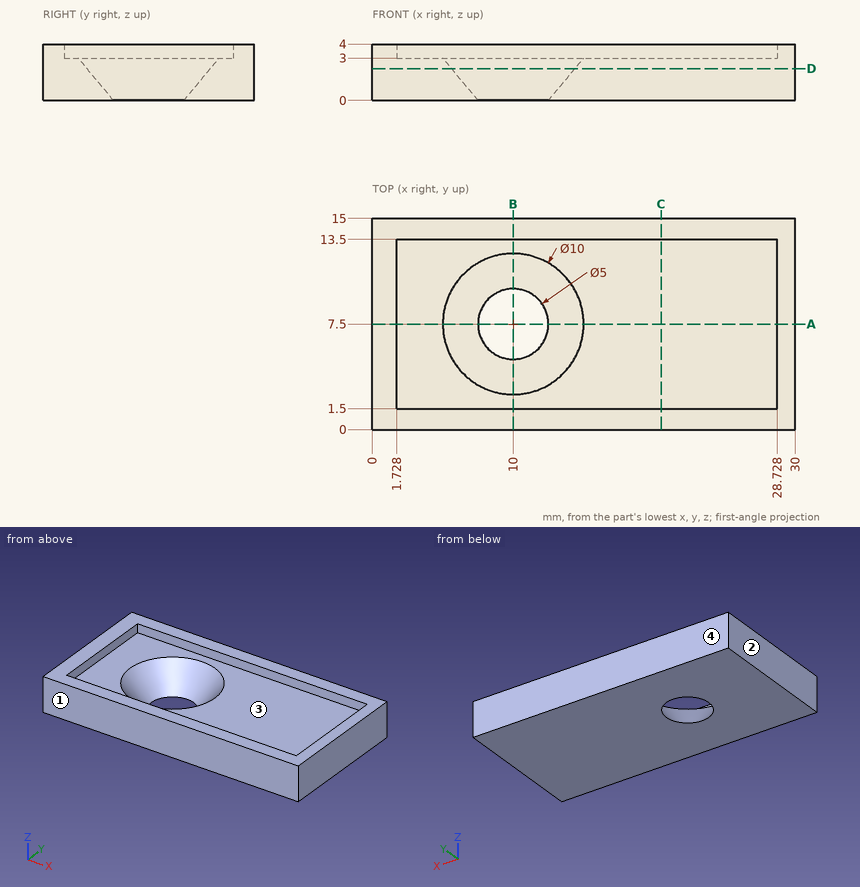
Geometry: see drawing. Coordinates: mm, zero at the bounding-box minimum. Give positions to 0.01 mm unless a question says otherwise; leave off trailing zeros. Order: outer loops, then holes, each group sorted by start corner. A loop starts at its lowest first (then second) coordinate and runs counter-clockwise, first axis right, second up. Notation, with made-up numbers: (77.5, -17) - (112.5, -17) arc R17 ccw to (112.5, 12) - close; hole circle Ø2 at (-22, 54.5). An arc over 180 degrees is marked (long way). Use CSV: the item, a comma, the result in double quotes.
1. Mould query, pull axis Y, two halves, no side actions, for the marked faces 1, 2, 3 and 4. Classes: +Y half, -Y half, draft (parallel to the pull), parting line (faces both ways), or undercut.
Answers below:
face 1,"-Y half"
face 2,"draft"
face 3,"undercut"
face 4,"+Y half"
2. Material intervals for line 1 along Y through (x, z) = (3.75, 3.4); line 2 along X through (y, z) = (9.5, 3.45); line 3 along Z through (x, y) = (27.25, 6.5), sorted ascending. Write a range as from..to.
Answers below:
line 1,"0..1.5, 13.5..15"
line 2,"0..1.73, 28.73..30"
line 3,"0..3"
3. Section query B-B (x = 10). Output: boundary loops of the cut face in (y, z), plus the area to 3 significant figures.
Answers below:
outline,"(0, 0) - (5, 0) - (2.5, 3) - (1.5, 3) - (1.5, 4) - (0, 4) - close; (10, 0) - (15, 0) - (15, 4) - (13.5, 4) - (13.5, 3) - (12.5, 3) - close"
area,"25.5 mm2"
4. Section query A-A (y = 7.5). Output: boundary loops of the cut face in (x, z).
Answers below:
outline,"(0, 0) - (7.5, 0) - (5, 3) - (1.73, 3) - (1.73, 4) - (0, 4) - close; (12.5, 0) - (30, 0) - (30, 4) - (28.73, 4) - (28.73, 3) - (15, 3) - close"
5. Section query C-C (x = 20.5). Output: boundary loops of the cut face in (y, z).
Answers below:
outline,"(0, 0) - (15, 0) - (15, 4) - (13.5, 4) - (13.5, 3) - (1.5, 3) - (1.5, 4) - (0, 4) - close"
6. Section query D-D (z = 2.25). Output: boundary loops of the cut face in (x, y) (3 decimals), plus the area to 3 significant figures.
Answers below:
outline,"(0, 0) - (30, 0) - (30, 15) - (0, 15) - close; hole circle Ø8.75 at (10, 7.5)"
area,"390 mm2"
7. Contact query for a flat-ended pin moving along its axis: pin 1 (3 mm diameter, centred on x = 16, y = 11, fed in from +Z). Output: stop coordinate, or through.
Answers below:
pin 1,"z = 3"
